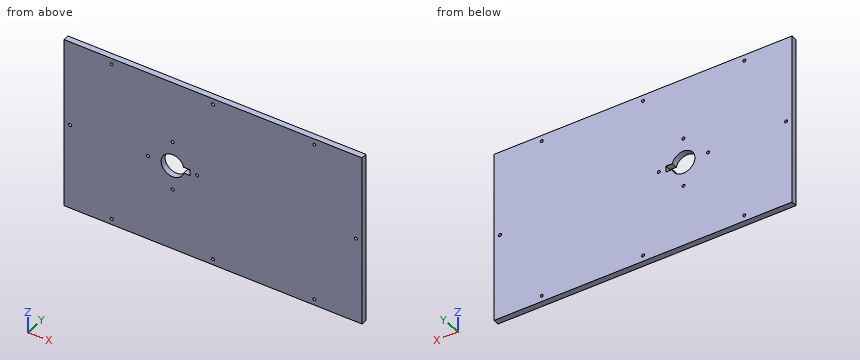
```python
from build123d import *

# Parameters (mm, degrees)
SKETCH1_W           = 500
SKETCH1_H           = 290
SKETCH1_R           = 2.5
BOSS_EXTRUDE1_DEPTH = 10


with BuildPart() as part:
    # Sketch1 → Boss-Extrude1 (new body)
    with BuildSketch(Plane(origin=(0, 0, 0), x_dir=(1, 0, 0), z_dir=(0, 1, 0))):
        Rectangle(SKETCH1_W, SKETCH1_H)
        with Locations((-240, 0)):
            Circle(SKETCH1_R, mode=Mode.SUBTRACT)
        with Locations((-170, -135)):
            Circle(SKETCH1_R, mode=Mode.SUBTRACT)
        with Locations((-170, 135)):
            Circle(SKETCH1_R, mode=Mode.SUBTRACT)
        with Locations((170, 135)):
            Circle(SKETCH1_R, mode=Mode.SUBTRACT)
        with Locations((240, 0)):
            Circle(SKETCH1_R, mode=Mode.SUBTRACT)
        with Locations((170, -135)):
            Circle(SKETCH1_R, mode=Mode.SUBTRACT)
        with Locations((0, 135)):
            Circle(SKETCH1_R, mode=Mode.SUBTRACT)
        with Locations((0, -135)):
            Circle(SKETCH1_R, mode=Mode.SUBTRACT)
        with Locations((-26.530336654, 0)):
            Circle(SKETCH1_R, mode=Mode.SUBTRACT)
        with Locations((-67.780336654, -41.25)):
            Circle(SKETCH1_R, mode=Mode.SUBTRACT)
        with Locations((-109.030336654, 0)):
            Circle(SKETCH1_R, mode=Mode.SUBTRACT)
        with Locations((-67.780336654, 41.25)):
            Circle(SKETCH1_R, mode=Mode.SUBTRACT)
        with BuildLine():
            Line((-49.191025209, -5), (-38.530336654, -5))
            Line((-38.530336654, -5), (-38.530336654, 5))
            Line((-38.530336654, 5), (-49.191025209, 5))
            ThreePointArc((-49.191025209, 5), (-87.030336654, 0), (-49.191025209, -5))
        make_face(mode=Mode.SUBTRACT)
    extrude(amount=BOSS_EXTRUDE1_DEPTH)


solid = part.part
```
Check sheet for the modelled part. Datum: model origin and axes. Units: mm. Round coordinates to 2 decimals unless told otherwise and drop trailing zeros. Loops run counter-clockwise (first coordinate to the right, second up) from the corner with the lowest first, then second, coordinate; pieces in that order, holes last. Notation, with made-up numbers: M 18.5,3.5 L 43.5,3.5 A26 cw 43.5,36.5 Z; hole C -12.5,36.25 d2. An arc over 180 degrees is marked long. Answer as a JSON object with one key per item and string values.
1. Section check A-A (z = -12). Record the boundary of the cut face in (x, y), plus the area to 3 significant figures.
Reply:
{"outline": "M -250,0 L -82.83,0 L -82.83,10 L -250,10 Z; M -52.73,0 L 250,0 L 250,10 L -52.73,10 Z", "area": "4,700 mm²"}
2. Gauge pin test, flat end, axial feed: P1, Ø23, axis at x = -67.78, z = 0, coming from the -Y side. Record the tip position at first contact, or that the pin passes through.
Reply:
{"P1": "passes through"}
3. Scan lines: line 1 (X direction, y = 5, z = 135); line 2 (Z direction, x = 0, y = 2.5); line 3 (X direction, y = 2, z = 0). Record each from-to range of solid material in increasing order.
Reply:
{"line 1": "x = -250 to -172.5, -167.5 to -2.5, 2.5 to 167.5, 172.5 to 250", "line 2": "z = -145 to -137.5, -132.5 to 132.5, 137.5 to 145", "line 3": "x = -250 to -242.5, -237.5 to -111.53, -106.53 to -87.03, -38.53 to -29.03, -24.03 to 237.5, 242.5 to 250"}
